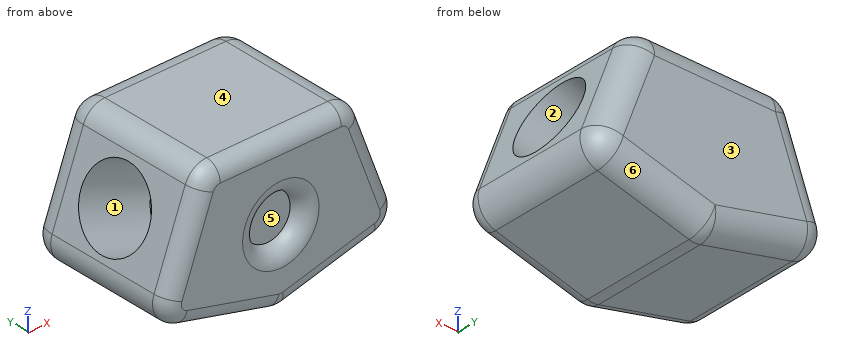
from build123d import *

# Parameters (mm, degrees)
BOSS_EXTRUDE1_DEPTH = 10
SKETCH2_R           = 2.5
CUT_EXTRUDE1_DEPTH  = 5
SKETCH3_R           = 2.5
CUT_EXTRUDE2_DEPTH  = 5
SKETCH4_R           = 1.5
CUT_EXTRUDE3_DEPTH  = 1
FILLET1_R           = 1.5
FILLET2_R           = 1.5
FILLET3_R           = 1


with BuildPart() as part:
    # Sketch1 → Boss-Extrude1 (new body)
    with BuildSketch(Plane(origin=(0, 0, 0), x_dir=(1, 0, 0), z_dir=(0, 1, 0))):
        Polygon((-5, 0), (5, 0), (8, 8), (0, 10), (-8, 8), align=None)
    extrude(amount=BOSS_EXTRUDE1_DEPTH)

    # Sketch2 → Cut-Extrude1 (cut)
    with BuildSketch(Plane(origin=(4.383561644, 0, 1.643835616), x_dir=(0.35112344158839154, 0, -0.9363291775690447), z_dir=(0.9363291775690445, 0, 0.3511234415883915))):
        with Locations((5.755617208, 5)):
            Circle(SKETCH2_R)
    extrude(amount=-CUT_EXTRUDE1_DEPTH, mode=Mode.SUBTRACT)

    # Sketch3 → Cut-Extrude2 (cut)
    with BuildSketch(Plane(origin=(-4.383561644, 0, 1.643835616), x_dir=(0.3511234415883919, 0, 0.9363291775690445), z_dir=(-0.9363291775690445, 0, 0.3511234415883919))):
        with Locations((-5.755617208, 5)):
            Circle(SKETCH3_R)
    extrude(amount=-CUT_EXTRUDE2_DEPTH, mode=Mode.SUBTRACT)

    # Sketch4 → Cut-Extrude3 (cut)
    with BuildSketch(Plane.XZ):
        with Locations(Location((0, -5, 0), (0, 0, 270))):
            Circle(SKETCH4_R)
    extrude(amount=-CUT_EXTRUDE3_DEPTH, mode=Mode.SUBTRACT)

    # Fillet1
    fillet1_edges = [part.edges().sort_by_distance(p)[0] for p in [
        (-8, 5, -8),
        (0, 5, -10),
        (8, 5, -8),
        (5, 5, 0),
        (-5, 5, 0),
    ]]
    fillet(fillet1_edges, radius=FILLET1_R)

    # Fillet2
    fillet2_edges = [part.edges().sort_by_distance(p)[0] for p in [
        (-3.366403469, 10, -9.158399133),
        (3.366403469, 10, -9.158399133),
        (-6.387343447, 10, -3.699582525),
        (0, 10, 0),
        (6.387343447, 10, -3.699582525),
        (7.333243577, 10, -7.649887814),
        (4.814891554, 10, -0.267111574),
        (-4.814891554, 10, -0.267111574),
        (-7.333243577, 10, -7.649887814),
        (0, 10, -9.95383539),
    ]]
    fillet(fillet2_edges, radius=FILLET2_R)

    # Fillet3
    fillet3_edges = [part.edges().sort_by_distance(p)[0] for p in [
        (0, 0, -3.5),
        (-3.366403469, 0, -9.158399133),
        (-6.387343447, 0, -3.699582525),
        (3.366403469, 0, -9.158399133),
        (6.387343447, 0, -3.699582525),
        (0, 0, 0),
        (7.333243577, 0, -7.649887814),
        (4.814891554, 0, -0.267111574),
        (-4.814891554, 0, -0.267111574),
        (-7.333243577, 0, -7.649887814),
        (0, 0, -9.95383539),
    ]]
    fillet(fillet3_edges, radius=FILLET3_R - 0.0001)  # a hair under: the kernel refuses the full size


solid = part.part
Can you work these out from the model? Positions are in its coordinate system, mm. Face numbers are marked on the shaded views. A direction names the side the tool comes from. Coordinates: 2 decimals unless noted, no trailing zeros. Loops run counter-clockwise (first coordinate to the right, second up) from the corner with the lowest first, then second, coordinate; pieces in that order, holes last. Notation, with made-up numbers: M 73,62 L 107,62 A21 cw 107,71 Z; hole C 79,16.25 d9. An arc over 180 degrees is marked long. Return JSON: item names as keys, results as strings. Group by question number.
Item 1: Thinking about a two-plate mould opening in Y: for the marked faces 1, 2, 3 and 4, which applies, released by +Y, released by -Y, zero draft, split by the parting line, or undercut?
Item 2: Imagine slicing it at B-B (y = 5.75). Please give me the cut outline in (x, z) (1 decimal), and give its area (3 significant figures).
Item 3: If I drill on L1, parallel to Y at x = -0.5, z = -5.75; L2, parallel to Y at x = -4.25, z = -2.75; L3, parallel to Y at x = 5, z = -2.75, over which ranges is the centre line in solid material (lowest first)? Write a range as from..to.
Item 4: Imagine slicing it at A-A (y = 8). Please give me the cut outline in (x, z) (1 decimal), and give its area (3 significant figures).
Item 5: I'm going to push a flat-ended pin straight in: pin 1 Ø0.9 at (x, z) = (0, -5.5) entering from -Y. Where does the tip first touch, or does it pass through?
Item 6: On a 3-axis mill with a long thin cutter (end or side, diameter ignored), from which of +Z, -Z, +X, -X, +Y, -Y can I reach the whole of each face in a straight line? I mean the marked faces 5 and 6. Say none if no direction works.
Verdict:
{
 "1": {"face 1": "undercut", "face 2": "undercut", "face 3": "released by +Y", "face 4": "zero draft"},
 "2": {"outline": "M -7.4,-6.4 A1.5 ccw -6.4,-8.4 L -0.4,-9.9 A1.5 ccw 0.4,-9.9 L 6.4,-8.4 A1.5 ccw 7.4,-6.4 L 7.2,-6 L 2.6,-7.7 L 0.9,-3.3 L 5.6,-1.5 L 5.4,-1 A1.5 ccw 4,0 L -4,0 A1.5 ccw -5.4,-1 L -5.6,-1.5 L -0.9,-3.3 L -2.6,-7.7 L -7.2,-6 Z", "area": "70.6 mm^2"},
 "3": {"L1": "y = 1..10", "L2": "y = 0..3.16, 6.84..10", "L3": "y = 0..2.95, 7.05..9.9"},
 "4": {"outline": "M -7.4,-6.4 A1.5 ccw -6.4,-8.4 L -0.4,-9.9 A1.5 ccw 0.4,-9.9 L 6.4,-8.4 A1.5 ccw 7.4,-6.4 L 5.4,-1 A1.5 ccw 4,0 L -4,0 A1.5 ccw -5.4,-1 Z", "area": "118 mm^2"},
 "5": {"pin 1": "stops at y = 1"},
 "6": {"face 5": "-Y", "face 6": "-Z, +X, +Y"}
}
